CAD build for the part. Positions are in the model's coordinates, mm. Give positions to 0.01 mm unless a question says otherwise; leave off trailing zeros. Loops run counter-clockwise (first coordinate to the right, second up) from the corner with the lowest first, then second, coordinate; pieces in that order, holes last. Notation, with made-up numbers: M 51,-25.75 L 110,-25.75 A14 cw 110,-10.75 Z; hole C -35,59.5 d6. An arc over 180 degrees is marked long. One line per question, with ' | ' between items.
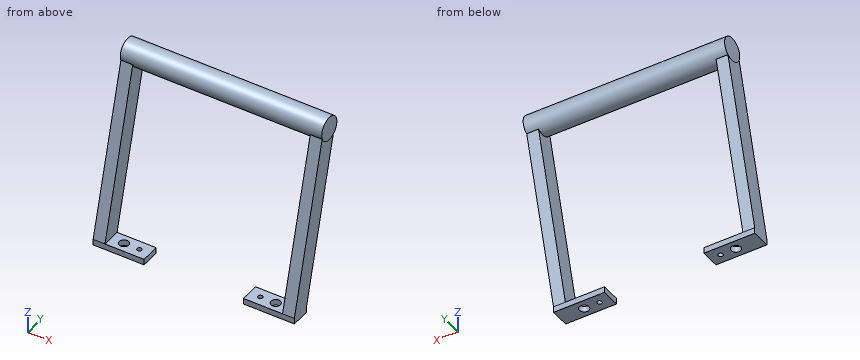
```python
from build123d import *

# Parameters (mm, degrees)
CYLINDER127_R             = 10
CYLINDER127_DEPTH         = 170.2
EXTRUDE010_DEPTH          = 10
FILLET003_R               = 7.72
FILLET003_ROLL_ANGLE      = 90
FILLET003_PLACEMENT_ANGLE = 90
EXTRUDE009_DEPTH          = 10
FILLET002_R               = 7.72
FILLET002_ROLL_ANGLE      = 90
FILLET002_PLACEMENT_ANGLE = 90
CYLINDER237_R             = 2
CYLINDER237_DEPTH         = 42
CYLINDER033_R             = 4
CYLINDER033_DEPTH         = 32
BOX309_W                  = 43
BOX309_H                  = 16
BOX309_DEPTH              = 5
CYLINDER236_R             = 2
CYLINDER236_DEPTH         = 42
CYLINDER034_R             = 4
CYLINDER034_DEPTH         = 32
BOX310_W                  = 43
BOX310_H                  = 16
BOX310_DEPTH              = 5


with BuildPart() as cylinder127:
    # Cylinder127 → Cylinder127 (new body)
    with BuildSketch(Plane(origin=(-119.1, 28, 146.3), x_dir=(0, 0, -1), z_dir=(1, 0, 0))):
        Circle(CYLINDER127_R)
    extrude(amount=CYLINDER127_DEPTH)


with BuildPart() as fillet003:
    # Wire005 → Extrude010 (new body)
    with BuildSketch(Plane.XY):
        Polygon((0, 0), (16, 0), (56, 150), (40, 150), align=None)
    extrude(amount=EXTRUDE010_DEPTH)

    # Fillet003
    fillet003_edges = [fillet003.edges().sort_by_distance(p)[0] for p in [
        (56, 150, 5),
        (40, 150, 5),
    ]]
    fillet(fillet003_edges, radius=FILLET003_R)


with BuildPart() as fillet003_1:
    # Fillet003 roll: moved
    add(fillet003.part.rotate(Axis((0, 0, 0), (1, 0, 0)), FILLET003_ROLL_ANGLE))


with BuildPart() as fillet003_2:
    # Fillet003 placement: moved
    add(fillet003_1.part.moved(Location((-119, -18, 5))).rotate(Axis((-119, -18, 5), (0, 0, 1)), FILLET003_PLACEMENT_ANGLE))


with BuildPart() as fusion167:
    # Wire004 → Extrude009 (new body)
    with BuildSketch(Plane.XY):
        Polygon((0, 0), (16, 0), (56, 150), (40, 150), align=None)
    extrude(amount=EXTRUDE009_DEPTH)

    # Fillet002
    fillet002_edges = [fusion167.edges().sort_by_distance(p)[0] for p in [
        (56, 150, 5),
        (40, 150, 5),
    ]]
    fillet(fillet002_edges, radius=FILLET002_R)


with BuildPart() as fusion167_1:
    # Fillet002 roll: moved
    add(fusion167.part.rotate(Axis((0, 0, 0), (1, 0, 0)), FILLET002_ROLL_ANGLE))


with BuildPart() as fusion167_2:
    # Fillet002 placement: moved
    add(fusion167_1.part.moved(Location((41, -18, 5))).rotate(Axis((41, -18, 5), (0, 0, 1)), FILLET002_PLACEMENT_ANGLE))

    # Fusion167: union Cylinder127, Fillet003
    add(cylinder127.part)
    add(fillet003_2.part)


with BuildPart() as cylinder237:
    # Cylinder237 → Cylinder237 (new body)
    with BuildSketch(Plane(origin=(17.2, -10, -5), x_dir=(1, 0, 0), z_dir=(0, 0, 1))):
        Circle(CYLINDER237_R)
    extrude(amount=CYLINDER237_DEPTH)


with BuildPart() as cylinder033:
    # Cylinder033 → Cylinder033 (new body)
    with BuildSketch(Plane(origin=(30.2, -10, 0), x_dir=(1, 0, 0), z_dir=(0, 0, 1))):
        Circle(CYLINDER033_R)
    extrude(amount=CYLINDER033_DEPTH)


with BuildPart() as cut203:
    # Box309 → Box309 (new body)
    with BuildSketch(Plane(origin=(8, -18, 0), x_dir=(1, 0, 0), z_dir=(0, 0, 1))):
        with Locations((21.5, 8)):
            Rectangle(BOX309_W, BOX309_H)
    extrude(amount=BOX309_DEPTH)

    # Cut187: cut Cylinder033
    add(cylinder033.part, mode=Mode.SUBTRACT)

    # Cut203: cut Cylinder237
    add(cylinder237.part, mode=Mode.SUBTRACT)


with BuildPart() as cylinder236:
    # Cylinder236 → Cylinder236 (new body)
    with BuildSketch(Plane(origin=(-85, -10, -5), x_dir=(1, 0, 0), z_dir=(0, 0, 1))):
        Circle(CYLINDER236_R)
    extrude(amount=CYLINDER236_DEPTH)


with BuildPart() as cylinder034:
    # Cylinder034 → Cylinder034 (new body)
    with BuildSketch(Plane(origin=(-98, -10, 0), x_dir=(1, 0, 0), z_dir=(0, 0, 1))):
        Circle(CYLINDER034_R)
    extrude(amount=CYLINDER034_DEPTH)


with BuildPart() as handle:
    # Box310 → Box310 (new body)
    with BuildSketch(Plane(origin=(-119, -18, 0), x_dir=(1, 0, 0), z_dir=(0, 0, 1))):
        with Locations((21.5, 8)):
            Rectangle(BOX310_W, BOX310_H)
    extrude(amount=BOX310_DEPTH)

    # Cut183: cut Cylinder034
    add(cylinder034.part, mode=Mode.SUBTRACT)

    # Cut202: cut Cylinder236
    add(cylinder236.part, mode=Mode.SUBTRACT)

    # Fusion169: union Fusion167, Cut203
    add(fusion167_2.part)
    add(cut203.part)


with BuildPart() as handle_1:
    # Fusion169 placement: moved
    add(handle.part.moved(Location((0, 0, 20.1))))


solid = handle_1.part
```
Item 1: Saw through at C-C on y = -10. Give the cut face in (x, z).
Conclusion:
outline: M -119,20.1 L -102,20.1 L -102,25.1 L -109,25.1 L -109,55.1 L -119,55.1 Z; M -94,20.1 L -87,20.1 L -87,25.1 L -94,25.1 Z; M -83,20.1 L -76,20.1 L -76,25.1 L -83,25.1 Z; M 8,20.1 L 15.2,20.1 L 15.2,25.1 L 8,25.1 Z; M 19.2,20.1 L 26.2,20.1 L 26.2,25.1 L 19.2,25.1 Z; M 34.2,20.1 L 51,20.1 L 51,55.1 L 41,55.1 L 41,25.1 L 34.2,25.1 Z
Item 2: Saw through at D-D on z = 145.5. Give the cut face in (x, y).
Conclusion:
outline: M -119,14.11 L -109,14.11 L -109,30.11 L -119,30.11 Z; M 41,14.11 L 51,14.11 L 51,30.11 L 41,30.11 Z
Item 3: Saw through at A-A on y = 9. Give the cut face in (x, z), and give its area (3 significant figures).
Conclusion:
outline: M -119,66.35 L -109,66.35 L -109,126.35 L -119,126.35 Z; M 41,66.35 L 51,66.35 L 51,126.35 L 41,126.35 Z | area: 1,200 mm²
Item 4: Drill centre lines: line 1 along X through (y, z) = (-10, 22.65); line 2 along Y through (x, z) = (-98, 21.3); line 3 along Y through (x, z) = (17.2, 21.5). Where is each one in solid material? Low to high. Write a range as [from, to].
Conclusion:
line 1: [-119, -102], [-94, -87], [-83, -76], [8, 15.2], [19.2, 26.2], [34.2, 51] | line 2: [-18, -14], [-6, -2] | line 3: [-18, -12], [-8, -2]
Item 5: Drop flat-ended pins along their axis: P1, Ø6.5, axis at x = 17.2, y = -10, coming from the -Z side; P2, Ø13, axis at x = 22, y = -9, coming from the +Z side; P3, Ø1.5, axis at x = 33, z = 21.5, coming from the +Y side; P4, Ø5, axis at y = 7.5, z = 106, coming from the -X side. Give the stop position or say it passes through.
Conclusion:
P1: z = 20.1 | P2: z = 25.1 | P3: y = -2 | P4: x = -119
Item 6: Saw through at B-B on x = 30.2. Give the cut face in (y, z).
Conclusion:
outline: M -18,20.1 L -14,20.1 L -14,25.1 L -18,25.1 Z; M -6,20.1 L -2,20.1 L -2,25.1 L -6,25.1 Z; C 28,166.4 d20
